from build123d import *
from build123d import SkipClean  # not in build123d's __all__

# Parameters (mm, degrees)
F0_W           = 87
F0_H           = 87
F0_R           = 2
F1_DEPTH       = 4
F2_R           = 4
F5_DEPTH       = 43.5
F6_T1_DEPTH    = 87
F7_R           = 20.025
F8_DEPTH       = 87.001
F9_R           = 2
F10_DEPTH      = 40.501
F11_R          = 20
F12_DEPTH      = 10
F15_DEPTH      = 106.5
F15_DEPTH_BACK = 25.4
F16_R          = 20
F17_DEPTH      = 150.0010001
F18_R          = 20
F19_DEPTH      = 15


# Not quite as in the source:
# - a fillet or chamfer that OpenCascade refuses, or shapes differently, is made with other operations: its cross-section is extruded or revolved along the edge and cut away or added
# - after a boolean that leaves OpenCascade's solid faulty, fix() repairs it


with BuildPart() as f1:
    # F0 (on Front) → F1 (new body)
    with BuildSketch(Plane.XZ):
        Rectangle(F0_W, F0_H)
        with Locations((-37.5, -37.5)):
            Circle(F0_R, mode=Mode.SUBTRACT)
        with Locations((37.5, -37.5)):
            Circle(F0_R, mode=Mode.SUBTRACT)
        with Locations((-37.5, 37.5)):
            Circle(F0_R, mode=Mode.SUBTRACT)
        with Locations((37.5, 37.5)):
            Circle(F0_R, mode=Mode.SUBTRACT)
    extrude(amount=F1_DEPTH)

    # F2
    f2_edges = [f1.edges().sort_by_distance(p)[0] for p in [
        (43.5, -2, 43.5),
        (-43.5, -2, 43.5),
        (43.5, -2, -43.5),
        (-43.5, -2, -43.5),
    ]]
    fillet(f2_edges, radius=F2_R)

    # F4 (on Top) → F5 (join, symmetric)
    with BuildSketch(Plane.XY):
        with BuildLine():
            ThreePointArc((-10.0623058987, 0), (-17.7800410903, 6.9119836686), (-21.3690774705, 16.6309225295))
            Line((-21.3690774705, 16.6309225295), (-38, 0))
            Line((-38, 0), (-10.0623058987, 0))
        make_face()
        with BuildLine():
            Line((-38, 0), (-21.3690774705, 16.6309225295))
            ThreePointArc((-21.3690774705, 16.6309225295), (-21.4314768317, 17.2848321331), (-21.4738707868, 17.9403427756))
            Line((-21.4738707868, 17.9403427756), (-39.4142135624, 0))
            Line((-39.4142135624, 0), (-38, 0))
        make_face()
        with BuildLine():
            ThreePointArc((-21.4738707868, 17.9403427756), (-21.4314768317, 17.2848321331), (-21.3690774705, 16.6309225295))
            ThreePointArc((-21.3690774705, 16.6309225295), (-17.7800410903, 6.9119836686), (-10.0623058987, 0))
            Line((-10.0623058987, 0), (10.0623058987, 0))
            ThreePointArc((10.0623058987, 0), (17.7800410903, 6.9119836686), (21.3690774705, 16.6309225295))
            ThreePointArc((21.3690774705, 16.6309225295), (21.4314768317, 17.2848321331), (21.4738707868, 17.9403427756))
            Line((21.4738707868, 17.9403427756), (19.9956189847, 19.4185945777))
            ThreePointArc((19.9956189847, 19.4185945777), (13.9933575036, 33.2893647786), (0, 39))
            ThreePointArc((0, 39), (-13.9933575036, 33.2893647786), (-19.9956189847, 19.4185945777))
            Line((-19.9956189847, 19.4185945777), (-21.4738707868, 17.9403427756))
        make_face()
        with BuildLine():
            ThreePointArc((21.5, 19), (-0.5299896624, 40.493466704), (-21.4738707868, 17.9403427756))
            Line((-21.4738707868, 17.9403427756), (-19.9956189847, 19.4185945777))
            ThreePointArc((-19.9956189847, 19.4185945777), (-13.9933575036, 33.2893647786), (0, 39))
            ThreePointArc((0, 39), (13.9933575036, 33.2893647786), (19.9956189847, 19.4185945777))
            Line((19.9956189847, 19.4185945777), (21.4738707868, 17.9403427756))
            ThreePointArc((21.4738707868, 17.9403427756), (21.493466704, 18.4700103376), (21.5, 19))
        make_face()
        with BuildLine():
            Line((10.0623058987, 0), (-10.0623058987, 0))
            ThreePointArc((-10.0623058987, 0), (0, -2.5), (10.0623058987, 0))
        make_face()
        with BuildLine():
            ThreePointArc((21.3690774705, 16.6309225295), (17.7800410903, 6.9119836686), (10.0623058987, 0))
            Line((10.0623058987, 0), (38, 0))
            Line((38, 0), (21.3690774705, 16.6309225295))
        make_face()
        with BuildLine():
            Line((39.4142135624, 0), (21.4738707868, 17.9403427756))
            ThreePointArc((21.4738707868, 17.9403427756), (21.4314768317, 17.2848321331), (21.3690774705, 16.6309225295))
            Line((21.3690774705, 16.6309225295), (38, 0))
            Line((38, 0), (39.4142135624, 0))
        make_face()
    extrude(amount=F5_DEPTH, both=True)

    # F6: fillet of radius 80 on 2 edges, made by hand

    # F6_s2 → F6_t1 (join)
    with BuildSketch(Plane.XY.offset(-43.5)):
        with BuildLine():
            ThreePointArc((-36.5156161223, 2.89859744), (-26.9555540815, 14.444838104), (-19.7173340913, 27.5718572276))
            ThreePointArc((-19.7173340913, 27.5718572276), (-21.1511313524, 22.857413967), (-21.4738707868, 17.9403427756))
            Line((-21.4738707868, 17.9403427756), (-36.5156161223, 2.89859744))
        make_face()
        with BuildLine():
            ThreePointArc((19.7173340913, 27.5718572276), (26.9555540815, 14.444838104), (36.5156161223, 2.89859744))
            Line((36.5156161223, 2.89859744), (21.4738707868, 17.9403427756))
            ThreePointArc((21.4738707868, 17.9403427756), (21.1511313524, 22.857413967), (19.7173340913, 27.5718572276))
        make_face()
    extrude(amount=F6_T1_DEPTH)

    # F7 (on face) → F8 (cut, through all)
    with BuildSketch(Plane.XY.offset(43.5)):
        with Locations((0, 19)):
            Circle(F7_R)
    extrude(amount=-F8_DEPTH, mode=Mode.SUBTRACT)

    # F9 (on Front) → F10 (cut, through all)
    with BuildSketch(Plane.XZ):
        with BuildLine():
            Line((-37.5, 35.5), (-37.5, 37.5))
            Line((-37.5, 37.5), (-35.5, 37.5))
            ThreePointArc((-35.5, 37.5), (-38.9142135624, 38.9142135624), (-37.5, 35.5))
        make_face()
        with BuildLine():
            Line((-35.5, 37.5), (-37.5, 37.5))
            Line((-37.5, 37.5), (-37.5, 35.5))
            ThreePointArc((-37.5, 35.5), (-36.0857864376, 36.0857864376), (-35.5, 37.5))
        make_face()
        with BuildLine():
            ThreePointArc((39.5, 37.5), (37.5, 39.5), (35.5, 37.5))
            ThreePointArc((35.5, 37.5), (37.5, 35.5), (39.5, 37.5))
        make_face()
        with BuildLine():
            ThreePointArc((-35.5, -37.5), (-36.0857864376, -36.0857864376), (-37.5, -35.5))
            ThreePointArc((-37.5, -35.5), (-38.9142135624, -38.9142135624), (-35.5, -37.5))
        make_face()
        with Locations((37.5, -37.5)):
            Circle(F9_R)
    with SkipClean():  # cleaning this boolean's faces spoils the solid; the shape is the same uncleaned
        extrude(amount=-F10_DEPTH, mode=Mode.SUBTRACT)

    # F14 (on Top) → F15 (join, two sides)
    with BuildSketch(Plane.XY) as f15_sk:
        with BuildLine():
            Line((-39.5, -4), (39.5, -4))
            Line((39.5, -4), (39.5, 0))
            Line((39.5, 0), (39.4142135624, 0))
            Line((39.4142135624, 0), (36.5156161223, 2.89859744))
            ThreePointArc((36.5156161223, 2.89859744), (26.9555540815, 14.444838104), (19.7173340913, 27.5718572276))
            ThreePointArc((19.7173340913, 27.5718572276), (0, 40.5), (-19.7173340913, 27.5718572276))
            ThreePointArc((-19.7173340913, 27.5718572276), (-26.9555540815, 14.444838104), (-36.5156161223, 2.89859744))
            Line((-36.5156161223, 2.89859744), (-39.4142135624, 0))
            Line((-39.4142135624, 0), (-39.5, 0))
            Line((-39.5, 0), (-39.5, -4))
        make_face()
    extrude(amount=F15_DEPTH)
    extrude(f15_sk.sketch, amount=-F15_DEPTH_BACK)

    add(f1.part.fix(), mode=Mode.REPLACE)

    # F16 (on face) → F17 (cut, through all)
    with BuildSketch(Plane.XY.offset(106.5)):
        with Locations((0, 19)):
            Circle(F16_R)
    extrude(amount=-F17_DEPTH, mode=Mode.SUBTRACT)

    # F18 (on face) → F19 (join)
    with BuildSketch(Plane.XY.offset(106.5)):
        with Locations((0, 19)):
            Circle(F18_R)
    extrude(amount=-F19_DEPTH)


with BuildPart() as f12:
    # F11 (on face) → F12 (new body)
    with BuildSketch(Plane(origin=(0, 0, -43.5), x_dir=(1, 0, 0), z_dir=(0, 0, -1))):
        with Locations((0, -19)):
            Circle(F11_R)
    extrude(amount=-F12_DEPTH)


solid = f1.part
The listing builds one solid part. Answer for the finished solid, in the listing's coordinates (mm). A direction names the side the tool comes from. Coordinates: 2 decimals unless noted, no trailing zeros. Loops run counter-clockwise (first coordinate to the right, second up) from the corner with the lowest first, then second, coordinate; pieces in that order, holes last. Notation, with made-up numbers: M 80.5,34 L 123.5,34 A24 ccw 123.5,50 Z; hole C 23.5,1 d1. An arc over 180 degrees is marked long. Answer in a Markdown table with one row per item.
1) Find section B-B (x = 0). Determine the outline of the cut face in (y, z) (3 decimals), then the cut area to 3 significant figures.
Answers below:
| item | result |
|---|---|
| outline | M -4,-43.5 L -1.025,-43.5 L -1.025,-25.4 L -1,-25.4 L -1,91.5 L 39,91.5 L 39,-25.4 L 39.025,-25.4 L 39.025,-43.5 L 40.5,-43.5 L 40.5,106.5 L -4,106.5 Z |
| area | 1,270 mm^2 |
2) Given pin 1 (4.5 mm diameter, centred on x = -42, z = 0, fed in from +Y); pin 2 (3 mm diameter, centred on y = -3, z = 62.5, fed in from -X); pin 3 (4.5 mm diameter, centred on x = 41, z = 11.5, fed in from +Y); pin 4 (2.5 mm diameter, centred on x = 37.5, z = -37.5, fed in from +Y), each flat-ended and moving along its own axis, determine where each tip first touches the part or whether it passes through.
Answers below:
| item | result |
|---|---|
| pin 1 | y = 0 |
| pin 2 | x = -39.5 |
| pin 3 | y = 0.66 |
| pin 4 | through |
3) Find section C-C (z = 96.5). Determine the outline of the cut face in (x, y).
Answers below:
| item | result |
|---|---|
| outline | M -39.5,-4 L 39.5,-4 L 39.5,0 L 39.41,0 L 36.52,2.9 A80 cw 19.72,27.57 A21.5 ccw -19.72,27.57 A80 cw -36.52,2.9 L -39.41,0 L -39.5,0 Z |
4) Which of the six approach directions +Z, -Z, +X, -X, +Y, -Y give full straight-line access (tool end or side, diameter ignored) to faces 5 (the cylindrical face through (35.502, -0.859, -37.412)), 6 (the flat face through (0, 19, 91.5)), 7 (the flat face through (39.5, -2, 75)), 8 (the flat face through (-43.5, -2, -1)), 9 (the flat face through (41, 0, -3))?
Answers below:
| item | result |
|---|---|
| face 5 | +Y, -Y |
| face 6 | -Z |
| face 7 | +Z, +X, +Y, -Y |
| face 8 | +Z, -Z, -X, +Y, -Y |
| face 9 | +Z, -Z, +X, +Y |
5) Determine the mould class of faces 1 (the flat face through (-41, 0, -3)), 2 (the cylindrical face through (-4.34, -0.55, -34.32)), 3 (the cylindrical face through (-42.359, -2.028, -42.297)), 4 (the cylindrical face through (-4.336, -0.524, 33.868)) for opening direction Y: released by +Y, released by -Y, zero draft, split by the parting line, or undercut.
Answers below:
| item | result |
|---|---|
| face 1 | released by +Y |
| face 2 | undercut |
| face 3 | zero draft |
| face 4 | undercut |
6) Find section A-A (z = 45). Determine the outline of the cut face in (x, y), then the cut area to 3 significant figures.
Answers below:
| item | result |
|---|---|
| outline | M -39.5,-4 L 39.5,-4 L 39.5,0 L 39.41,0 L 36.52,2.9 A80 cw 19.72,27.57 A21.5 ccw -19.72,27.57 A80 cw -36.52,2.9 L -39.41,0 L -39.5,0 Z; hole C 0,19 d40 |
| area | 978 mm^2 |
7) Find the intervals of material crossed by probe 1 along Y at (x, z) = (0, 67); probe 2 along X at (y, z) = (-1.5, -37.5); probe 3 along X at (y, z) = (15, 14), in increasing order.
Answers below:
| item | result |
|---|---|
| probe 1 | -4 to -1, 39 to 40.5 |
| probe 2 | -43.5 to -39.5, -35.5 to 35.5, 39.5 to 43.5 |
| probe 3 | -26.58 to -19.6, 19.6 to 26.58 |
